from build123d import *

# Parameters (mm, degrees)
BOSS_EXTRUDE1_DEPTH = 2


with BuildPart() as part:
    # Sketch1 → Boss-Extrude1 (new body)
    with BuildSketch(Plane.XY):
        Polygon((-481.45546786, 0), (478.54453214, 0), (478.54453214, 5), (448.54453214, 5), (448.54453214, 110), (436.54453214, 110), (436.54453214, 5), (411.54453214, 5), (411.54453214, 110), (399.54453214, 110), (399.54453214, 5), (374.54453214, 5), (374.54453214, 110), (362.54453214, 110), (362.54453214, 5), (337.54453214, 5), (337.54453214, 110), (325.54453214, 110), (325.54453214, 5), (300.54453214, 5), (300.54453214, 110), (288.54453214, 110), (288.54453214, 5), (263.54453214, 5), (263.54453214, 110), (251.54453214, 110), (251.54453214, 5), (226.54453214, 5), (226.54453214, 110), (214.54453214, 110), (214.54453214, 5), (189.54453214, 5), (189.54453214, 110), (177.54453214, 110), (177.54453214, 5), (152.54453214, 5), (152.54453214, 110), (140.54453214, 110), (140.54453214, 5), (115.54453214, 5), (115.54453214, 110), (103.54453214, 110), (103.54453214, 5), (78.54453214, 5), (78.54453214, 110), (66.54453214, 110), (66.54453214, 5), (41.54453214, 5), (41.54453214, 110), (29.54453214, 110), (29.54453214, 5), (4.54453214, 5), (4.54453214, 110), (-7.45546786, 110), (-7.45546786, 5), (-32.45546786, 5), (-32.45546786, 110), (-44.45546786, 110), (-44.45546786, 5), (-69.45546786, 5), (-69.45546786, 110), (-81.45546786, 110), (-81.45546786, 5), (-106.45546786, 5), (-106.45546786, 110), (-118.45546786, 110), (-118.45546786, 5), (-143.45546786, 5), (-143.45546786, 110), (-155.45546786, 110), (-155.45546786, 5), (-180.45546786, 5), (-180.45546786, 110), (-192.45546786, 110), (-192.45546786, 5), (-217.45546786, 5), (-217.45546786, 110), (-229.45546786, 110), (-229.45546786, 5), (-254.45546786, 5), (-254.45546786, 110), (-266.45546786, 110), (-266.45546786, 5), (-291.45546786, 5), (-291.45546786, 110), (-303.45546786, 110), (-303.45546786, 5), (-328.45546786, 5), (-328.45546786, 110), (-340.45546786, 110), (-340.45546786, 5), (-365.45546786, 5), (-365.45546786, 110), (-377.45546786, 110), (-377.45546786, 5), (-402.45546786, 5), (-402.45546786, 110), (-414.45546786, 110), (-414.45546786, 5), (-439.45546786, 5), (-439.45546786, 110), (-451.45546786, 110), (-451.45546786, 5), (-491.45546786, 5), (-491.45546786, 0), align=None)
    extrude(amount=BOSS_EXTRUDE1_DEPTH)


solid = part.part
Work out the finished part from the listing and answer in its coordinate system (mm). Coordinates: 2 decimals unless noted, no trailing zeros. Write each loop counter-clockwise with the first axis right and the second up, starting at its lowest first coordinate (ties: lowest second). Pieces come first, ordered by that corner, then holes. Notation, with made-up numbers: M -25.5,47 L -21.5,47 A7 ccw -21.5,59 Z; hole C 61.25,51.25 d9. An arc over 180 degrees is marked long. Use one line per item in the form item = value. Start each with the question number.
1. The part is cut by section A-A (y = 17). Give the number of separate pieces and of enclosed holes in the cut face, plus the area to 3 significant figures.
2. A straight line is drawn through the part: probe 1 along Y at (x, z) = (190, 1.35). Find the intervals that lie inside material, in ascending order. Write a range as from..to.
3. The part is cut by section B-B (x = 130). Give the vertices of the cut face in (y, z).
4. Each of these flat-tipped pins is pushed along its axis until it touches: P1, Ø1, axis at y = 62, z = 0.5, coming from the -X side; P2, Ø1, axis at y = 80, z = 1, coming from the +X side; P3, Ø1, axis at x = 238.5, z = 0.5, coming from the +Y side. Where does it stop, or does it pass through?
Evaluation:
q1.separate_pieces = 25
q1.enclosed_holes = 0
q1.area = 600 mm^2
q2.probe_1 = 0..5
q3.outline = M 0,0 L 5,0 L 5,2 L 0,2 Z
q4.P1 = -451.46
q4.P2 = 448.54
q4.P3 = 5
